from build123d import *

# Parameters (mm, degrees)
F0_R     = 20
F1_DEPTH = 5
F2_R     = 1
F3_DEPTH = 7


with BuildPart() as f1:
    # F0 (on Front) → F1 (new body)
    with BuildSketch(Plane.XZ):
        with BuildLine():
            ThreePointArc((24.8746859277, -2.5), (24.9686518278, -1.2515693765), (25, 0))
            ThreePointArc((25, 0), (24.9686518278, 1.2515693765), (24.8746859277, 2.5))
            Line((24.8746859277, 2.5), (24.8746859277, -2.5))
        make_face()
        with BuildLine():
            ThreePointArc((24.8746859277, 2.5), (24.9686518278, 1.2515693765), (25, 0))
            ThreePointArc((25, 0), (24.9686518278, -1.2515693765), (24.8746859277, -2.5))
            Line((24.8746859277, -2.5), (29.8746859277, -2.5))
            Line((29.8746859277, -2.5), (29.8746859277, 2.5))
            Line((29.8746859277, 2.5), (24.8746859277, 2.5))
        make_face()
        with BuildLine():
            Line((24.8746859277, -2.5), (24.8746859277, 2.5))
            ThreePointArc((24.8746859277, 2.5), (17.6776695297, 17.6776695297), (2.5, 24.8746859277))
            Line((2.5, 24.8746859277), (-2.5, 24.8746859277))
            ThreePointArc((-2.5, 24.8746859277), (-17.6776695297, 17.6776695297), (-24.8746859277, 2.5))
            ThreePointArc((-24.8746859277, 2.5), (-25, 0), (-24.8746859277, -2.5))
            ThreePointArc((-24.8746859277, -2.5), (-17.6776695297, -17.6776695297), (-2.5, -24.8746859277))
            ThreePointArc((-2.5, -24.8746859277), (0, -25), (2.5, -24.8746859277))
            ThreePointArc((2.5, -24.8746859277), (17.6776695297, -17.6776695297), (24.8746859277, -2.5))
        make_face()
        Circle(F0_R, mode=Mode.SUBTRACT)
        with BuildLine():
            Line((-2.5, 24.8746859277), (2.5, 24.8746859277))
            ThreePointArc((2.5, 24.8746859277), (0, 25), (-2.5, 24.8746859277))
        make_face()
        with BuildLine():
            ThreePointArc((-2.5, 24.8746859277), (0, 25), (2.5, 24.8746859277))
            Line((2.5, 24.8746859277), (2.5, 29.8746859277))
            Line((2.5, 29.8746859277), (-2.5, 29.8746859277))
            Line((-2.5, 29.8746859277), (-2.5, 24.8746859277))
        make_face()
        with BuildLine():
            Line((2.5, -29.8746859277), (2.5, -24.8746859277))
            ThreePointArc((2.5, -24.8746859277), (0, -25), (-2.5, -24.8746859277))
            Line((-2.5, -24.8746859277), (-2.5, -29.8746859277))
            Line((-2.5, -29.8746859277), (2.5, -29.8746859277))
        make_face()
        with BuildLine():
            ThreePointArc((-24.8746859277, -2.5), (-25, 0), (-24.8746859277, 2.5))
            Line((-24.8746859277, 2.5), (-29.8746859277, 2.5))
            Line((-29.8746859277, 2.5), (-29.8746859277, -2.5))
            Line((-29.8746859277, -2.5), (-24.8746859277, -2.5))
        make_face()
    extrude(amount=F1_DEPTH)

    # F2 (on Front) → F3 (join)
    with BuildSketch(Plane.XZ):
        with Locations((0, 22.5)):
            Circle(F2_R)
        with Locations((0, -22.5)):
            Circle(F2_R)
        with Locations((22.5, 0)):
            Circle(F2_R)
        with Locations((-22.5, 0)):
            Circle(F2_R)
    extrude(amount=F3_DEPTH)


solid = f1.part
Here's how the part is built. I have some questions about the finished solid (model axes, mm). A direction names the side the tool comes from. Give positions to 0.01 mm unless a question says otherwise; leave off trailing zeros. Order: outer loops, then holes, each group sorted by start corner. A loop starts at its lowest first (then second) coordinate and runs counter-clockwise, first axis right, second up. Notation, with made-up numbers: (-31, 55) -> (-3, 55) arc R30 cw to (-3, 87) -> close; hole circle Ø6 at (29, 26). An arc over 180 degrees is marked (long way). One line per item, written item: value. Start each with the question number.
1. Will these pins go through, and if not, where does the flat tip stop? pin 1 Ø2.5 at (x, y) = (27.5, -1.5) entering from -Z; pin 2 Ø1.5 at (y, z) = (-2, -28.5) entering from +X; pin 3 Ø2.5 at (y, z) = (-2, -27.5) entering from -X.
2. Imagine slicing it at B-B, the plane x = 19. List the corners of the cut face in (y, z) for me (3 decimals), plus the area to 3 significant figures.
3. Imagine slicing it at C-C, the plane z = -10. List the corners of the cut face in (x, y) for me, plus the area to 3 significant figures.
4. Imagine slicing it at D-D, the plane x = -22.5. List the corners of the cut face in (y, z) for me, plus the area to 3 significant figures.
5. We'd pull the mould along X, two halves only. Please class faces 1 (the face through (17.507, -2.465, -17.846)), 2 (the face through (21.5, -6, 0)), 3 (the face through (27, -2, 2.5)): released by +X, released by -X, zero draft, split by the parting line, or undercut.
6. I need wall thicknesses on probe 1 along Z at (x, y) = (0, -2.1); probe 2 along Z at (x, y) = (-14, -3); probe 3 along Y at (x, z) = (19, -7.5). Which ranges of each line are inside material? Lowest first, please. Write a range as from..to.
7. Imagine slicing it at A-A, the plane y = -1. List the corners of the cut face in (x, z) for me, plus the area to 3 significant figures.
8. For faces 4 (the face through (27, -2, -2.5)), 5 (the face through (0, -2, -29.875)), 6 (the face through (-0.217, -5.986, -23.476)), 7 (the face through (2.5, -2, 27)), 8 (the face through (-2.5, -2, -27)), which set-ups out of +Z, -Z, +X, -X, +Y, -Y let a thin tool reach every point of the face, with its end or its side?
Values follow:
1. pin 1: stops at z = -2.5
1. pin 2: stops at x = 2.5
1. pin 3: stops at x = -2.5
2. outline: (-5, -16.248) -> (0, -16.248) -> (0, -6.245) -> (-5, -6.245) -> close; (-5, 6.245) -> (0, 6.245) -> (0, 16.248) -> (-5, 16.248) -> close
2. area: 100 mm2
3. outline: (-22.91, -5) -> (-17.32, -5) -> (-17.32, 0) -> (-22.91, 0) -> close; (17.32, -5) -> (22.91, -5) -> (22.91, 0) -> (17.32, 0) -> close
3. area: 55.9 mm2
4. outline: (-7, -1) -> (-5, -1) -> (-5, -10.9) -> (0, -10.9) -> (0, 10.9) -> (-5, 10.9) -> (-5, 1) -> (-7, 1) -> close
4. area: 113 mm2
5. face 1: released by +X
5. face 2: undercut
5. face 3: zero draft
6. probe 1: z = -29.87..-20, 20..29.87
6. probe 2: z = -20.71..-14.28, 14.28..20.71
6. probe 3: y = -5..0
7. outline: (-29.87, -2.5) -> (-24.87, -2.5) arc R25 ccw to (-2.5, -24.87) -> (-2.5, -29.87) -> (2.5, -29.87) -> (2.5, -24.87) arc R25 ccw to (24.87, -2.5) -> (29.87, -2.5) -> (29.87, 2.5) -> (24.87, 2.5) arc R25 ccw to (2.5, 24.87) -> (2.5, 29.87) -> (-2.5, 29.87) -> (-2.5, 24.87) arc R25 ccw to (-24.87, 2.5) -> (-29.87, 2.5) -> close; hole circle Ø40 at (0, 0)
7. area: 805 mm2
8. face 4: -Z, +X, +Y, -Y
8. face 5: -Z, +X, -X, +Y, -Y
8. face 6: -Y
8. face 7: +Z, +X, +Y, -Y
8. face 8: -Z, -X, +Y, -Y
